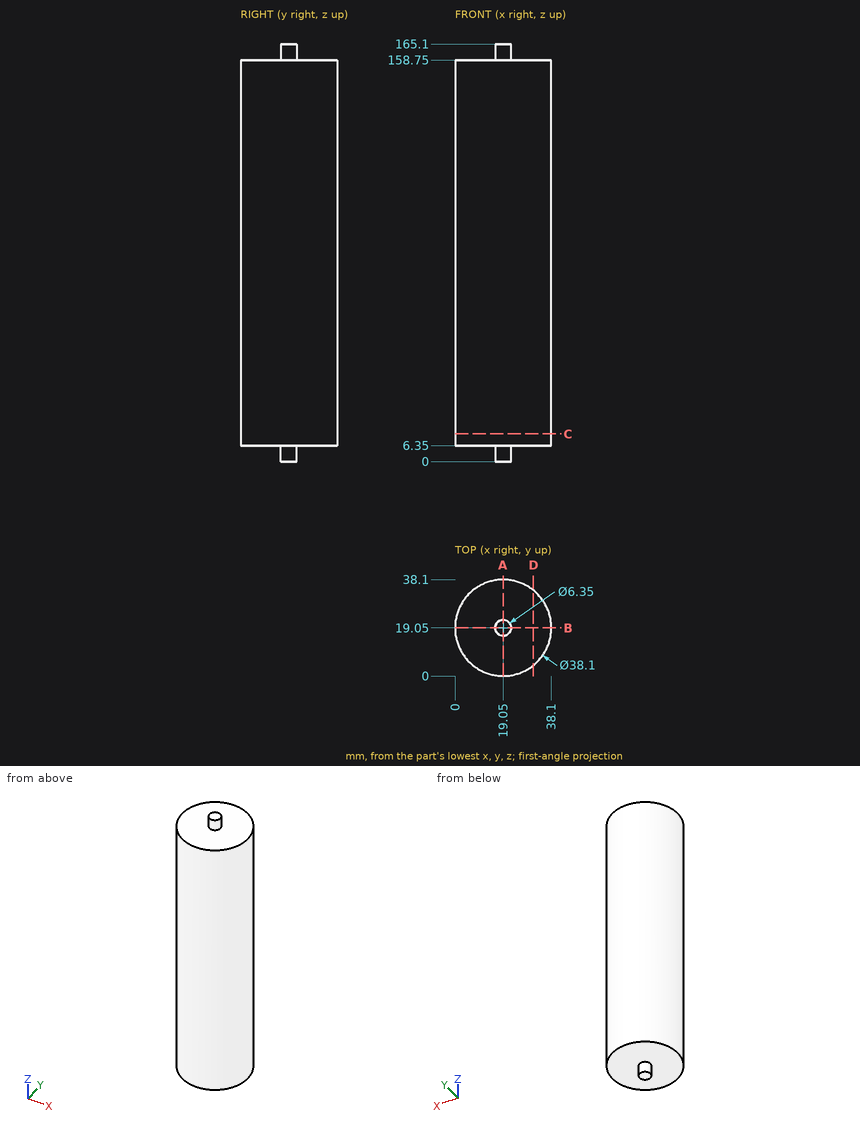
Part print with two shaded views. Sizes in mm from the minimum x, y, z corner. Coordinates: 2 decimals unless noted, no trailing zeros. Loops run counter-clockwise (first coordinate to the right, second up) from the corner with the lowest first, then second, coordinate; pieces in that order, holes last. Notation, with made-up numbers: (81.5, 10.25) - (135.5, 10.25) arc R15 ccw to (135.5, 28.25) - close; hole circle Ø1 at (41, -19). An arc over 180 degrees is marked (long way). Write each question's results on one line, items separated by ' | '. Start each with the question number.
Q1. Slice it at D-D on x = 31. Give the cut face in (y, z), and give its area (3 significant figures).
Q2. Slice it at A-A on x = 19.05. Give the cut face in (y, z) (3 decimals), and give its area (3 significant figures).
Q3. Probe line 1 along Z through (x, y) = (16, 8); line 2 along Y through (x, z) = (20, 26.5); line 3 along X through (y, z) = (22, 123.5). List the from-to ranges inside material, lowest first.
Q4. Slice it at C-C on z = 11. Give the cut face in (x, y).
Q5. Drop flat-ended pins along their axis: pin 1 Ø8 at (x, y) = (11, 33.5) entering from +Z; pin 2 Ø4 at (x, y) = (25, 12.5) entering from -Z; pin 3 Ø19 at (x, y) = (23.5, 15.5) entering from -Z; pin 4 Ø8 at (y, z) = (31.5, 103.5) entering from -X. Give the stop position or say it passes through.
Answer:
1) outline: (4.21, 6.35) - (33.89, 6.35) - (33.89, 158.75) - (4.21, 158.75) - close | area: 4,520 mm2
2) outline: (0, 6.35) - (15.875, 6.35) - (15.875, 0) - (22.225, 0) - (22.225, 6.35) - (38.1, 6.35) - (38.1, 158.75) - (22.225, 158.75) - (22.225, 165.1) - (15.875, 165.1) - (15.875, 158.75) - (0, 158.75) - close | area: 5,890 mm2
3) line 1: z = 6.35 to 158.75 | line 2: y = 0.02 to 38.08 | line 3: x = 0.23 to 37.87
4) outline: circle Ø38.1 at (19.05, 19.05)
5) pin 1: stops at z = 158.75 | pin 2: stops at z = 6.35 | pin 3: stops at z = 0 | pin 4: stops at x = 1.98
